Work out the finished part from the listing and answer in its coordinate system (mm). A direction names the side the tool comes from. Coordinates: 2 decimals unless noted, no trailing zeros. Order: outer loops, then holes, each group sorted by start corner. A loop starts at its lowest first (then second) coordinate and runs counter-clockwise, first axis right, second up. Notation, with made-up numbers: (40, 39.25) -> (91, 39.25) arc R25 ccw to (91, 51.25) -> close; hole circle Ø4 at (45.5, 10). An arc over 180 degrees is marked (long way). Write item = value, one per line. Start each with the question number.
Q1. Straight lines are drawn through the part: L1, parallel to Y at x = -25, z = 1.6 (3 decimals); L2, parallel to Y at x = -0.7, z = 28; L3, parallel to Z at x = -36, y = 448. For each, find the intervals that lie inside material, in ascending order. Write a range as from..to.
Q2. The part is cut by section B-B, the plane z = 9. Determine the outline of the cut face in (x, y).
Q3. Flat-ended cylindrical pins translate along their axes: pin 1 (6 mm diameter, centred on y = 149.26, z = 28, fed in from -X); pin 2 (15.5 mm diameter, centred on y = 59.26, z = 28, fed in from -X); pin 3 (1.5 mm diameter, centred on x = -22, y = 72.5, fed in from +Z). Find the tip coordinate at first contact, or state that the pin passes through.
Q4. The part is cut by section A-A, the plane y = 513.5. Determine the outline of the cut face in (x, z).
Q5. Which of the six approach directions +Z, -Z, +X, -X, +Y, -Y give full straight-line access (tool end or side, diameter ignored) to faces 1 (the flat face through (-2.7, 0, 14)), 2 (the flat face through (-26, 326, 3))?
Q6. The part is cut by section C-C, the plane x = -8.5. Determine the outline of the cut face in (y, z), plus the area to 3 significant figures.
Autodesk Inventor part; units mm, degrees
ref_plane "YZ Plane" through (0, 0, 0) normal (1, 0, 0) x (0, 1, 0)
ref_plane "XZ Plane" through (0, 0, 0) normal (0, 1, 0) x (-1, 0, 0)
ref_plane "XY Plane" through (0, 0, 0) normal (0, 0, 1) x (1, 0, 0)
sketch "Sketch1" plane through (0, 0, 0) normal (0, 1, 0) x (-1, 0, 0)
  line L0 (0, 0) -> (50, 0)
  line L1 (50, 0) -> (50, 3)
  line L2 (0, 0) -> (0, 50)
  line L3 (0, 50) -> (3, 50)
  line L4 (3, 50) -> (3, 3)
  line L5 (3, 3) -> (50, 3)
  dimension "d0" = 50
  dimension "d1" = 3
  dimension "d2" = 50
  dimension "d3" = 3
extrude "Extrusion1" add sketch "Sketch1" along normal blind 660.4
sketch "Sketch4" plane through (0, 0, 0) normal (0, 0, -1) x (-1, 0, 0)
  circle A0 centre (25, 15.7) radius 3.175
  circle A1 centre (25, 644.7) radius 3.175
  dimension "d62" = 6.35
  dimension "d63" = 6.35
extrude "Extrusion4" cut sketch "Sketch4" against normal blind 25.4
sketch "Sketch5" plane through (-3, 0, 3) normal (-1, 0, 0) x (0, 0, 1)
  circle A0 centre (25, 59.2629) radius 4.8387
  circle A1 centre (25, 149.2629) radius 4.8387
  circle A2 centre (25, 219.0371) radius 4.8387
  circle A3 centre (25, 309.0371) radius 4.8387
  line L0 (0, 0) -> (47, 0)
  line L1 (0, 0) -> (0, 660.4)
  line L2 (-136.6387, 184.15) -> (192.6114, 184.15) construction
  line L3 (47, 0) -> (47, 660.4)
  line L4 (-3, 0) -> (-3, 660.4) construction
  dimension "d68" = 90
  dimension "d70" = 90
  dimension "d71" = 69.7742
  dimension "d72" = 184.15
  dimension "d73" = 34.8871
  dimension "d74" = 34.8871
  dimension "d77" = 25
  dimension "d78" = 59.2629
  dimension "d79" = 50
extrude "Extrusion5" cut sketch "Sketch5" against normal blind 25.4
equation "\"d63\" = d62"
equation "\"d70\" = d68"
equation "\"d73\" = 0.5 * d71"
equation "\"d74\" = 0.5 * d71"
equation "\"d77\" = 0.5 * d79"
properties part number "26in Angle Channel CIM Mount Left" material "Aluminum 6061"
Model answer:
q1.L1 = 0..12.525, 18.875..641.525, 647.875..660.4
q1.L2 = 0..54.42, 64.1..144.42, 154.1..214.2, 223.88..304.2, 313.88..660.4
q1.L3 = 0..3
q2.outline = (-3, 0) -> (0, 0) -> (0, 660.4) -> (-3, 660.4) -> close
q3.pin_1 = through
q3.pin_2 = -3
q3.pin_3 = 3
q4.outline = (-50, 0) -> (0, 0) -> (0, 50) -> (-3, 50) -> (-3, 3) -> (-50, 3) -> close
q5.face_1 = +Z, -Z, +X, -X, -Y
q5.face_2 = +Z, -X, +Y, -Y
q6.outline = (0, 0) -> (660.4, 0) -> (660.4, 3) -> (0, 3) -> close
q6.area = 1,980 mm2
